```python
from build123d import *

# Parameters (mm, degrees)
SKETCH_1_R          = 10
EXTRUDE_1_DEPTH     = 2.5
SKETCH_2_R          = 4.5
SKETCH_2_R_2        = 3
EXTRUDE_2_DEPTH     = 2
SKETCH_3_R          = 1.25
CUT_EXTRUDE_1_DEPTH = 15.361406616


with BuildPart() as part:
    # 草图1 → 凸台-拉伸1 (new body)
    with BuildSketch(Plane.XY):
        Circle(SKETCH_1_R)
    extrude(amount=EXTRUDE_1_DEPTH)

    # 草图2 → 凸台-拉伸2 (add)
    with BuildSketch(Plane.XY.offset(2.5)):
        Circle(SKETCH_2_R)
        Circle(SKETCH_2_R_2, mode=Mode.SUBTRACT)
    extrude(amount=EXTRUDE_2_DEPTH)

    # 草图3 → 切除-拉伸1 (cut, through all)
    with BuildSketch(Plane.XY.offset(2.5)):
        with Locations((0, 7)):
            Circle(SKETCH_3_R)
        with Locations((7, 0)):
            Circle(SKETCH_3_R)
        with Locations((0, -7)):
            Circle(SKETCH_3_R)
        with Locations((-7, 0)):
            Circle(SKETCH_3_R)
    extrude(amount=-CUT_EXTRUDE_1_DEPTH, mode=Mode.SUBTRACT)


solid = part.part
```
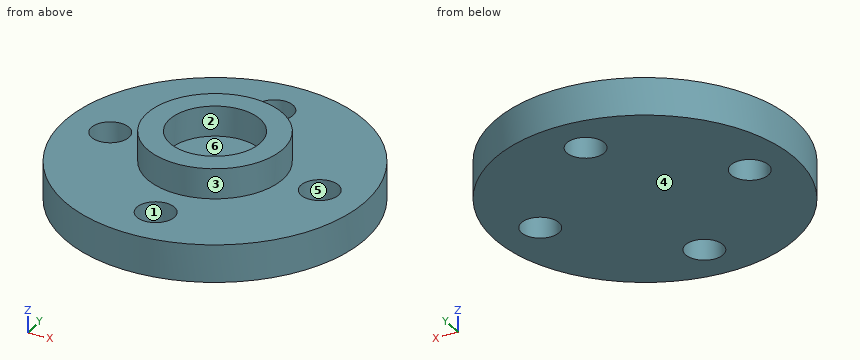
Verification items for the finished model (mm, model axes). Face numbers are marked on the shaded views. A direction names the side the tool comes from. Coordinates: 2 decimals unless noted, no trailing zeros. Write each loop counter-clockwise with the first axis right and the second up, starting at its lowest first coordinate (ties: lowest second). Pieces come first, ordered by that corner, then holes. Notation, with made-up numbers: M 70,-5 L 115,-5 A26 ccw 115,29 Z; hole C 63.5,80 d5. An arc over 180 degrees is marked long. Answer as a JSON object with one key per item and string values. Group by question number.
(1) Material ranges on line 1 (Y direction, x = 0, z = 0.65); line 2 (Y direction, x = 0, z = 3.4); line 3 (Z direction, x = 2.75, y = 6.25), recorded low to high.
(2) Cross-section at C-C, the plane y = -7. Record the cut outline in (x, z).
(3) Cross-section at D-D, the plane z = 0.6. Record the cut outline in (x, y).
(4) Tool access check on the marked faces 1 and 2. Record the directions out of +Z, -Z, +X, -X, +Y, -Y that give a thin tool (end or side, any length) a straight path to the whole face; none if there is none.
(5) Cross-section at A-A, the plane y = 0. Record the cut outline in (x, z).
(6) Release check for a two-part mould opening along Y. For the marked faces 3, 4, 5 and 6 record: +Y half, -Y half, draft (parallel to the pull), parting line (faces both ways), or undercut.
(7) Gauge pin test, flat ends, axial feed: pin 1 (4 mm diameter, centred on x = 7, y = 0, fed in from +Z); pin 2 (1.5 mm diameter, centred on x = 0, y = -7, fed in from +Z). Record the tip position at first contact, or that the pin passes through.
Reply:
{
 "1": {"line 1": "-10 to -8.25, -5.75 to 5.75, 8.25 to 10", "line 2": "-4.5 to -3, 3 to 4.5", "line 3": "0 to 2.5"},
 "2": {"outline": "M -7.14,0 L -1.25,0 L -1.25,2.5 L -7.14,2.5 Z; M 1.25,0 L 7.14,0 L 7.14,2.5 L 1.25,2.5 Z"},
 "3": {"outline": "C 0,0 d20; hole C -7,0 d2.5; hole C 0,-7 d2.5; hole C 0,7 d2.5; hole C 7,0 d2.5"},
 "4": {"face 1": "+Z, -Z", "face 2": "+Z"},
 "5": {"outline": "M -10,0 L -8.25,0 L -8.25,2.5 L -10,2.5 Z; M -5.75,0 L 5.75,0 L 5.75,2.5 L 4.5,2.5 L 4.5,4.5 L 3,4.5 L 3,2.5 L -3,2.5 L -3,4.5 L -4.5,4.5 L -4.5,2.5 L -5.75,2.5 Z; M 8.25,0 L 10,0 L 10,2.5 L 8.25,2.5 Z"},
 "6": {"face 3": "parting line", "face 4": "draft", "face 5": "undercut", "face 6": "undercut"},
 "7": {"pin 1": "z = 2.5", "pin 2": "through"}
}
